```python
from build123d import *

# Parameters (mm, degrees)
SKETCH1_W                       = 22.225
SKETCH1_H                       = 22.225
BOSS_EXTRUDE1_DEPTH             = 38.1
BOSS_EXTRUDE3_REACH             = 43.214
BOSS_EXTRUDE3_DIRECTION_2_REACH = 43.214
SKETCH4_R                       = 2.159
CUT_EXTRUDE1_DEPTH              = 46.486792383
SKETCH8_R                       = 1.5875
CUT_EXTRUDE3_DEPTH              = 8.89
SKETCH7_R                       = 1.5875
CUT_EXTRUDE4_DEPTH              = 8.89
CUT_EXTRUDE6_DEPTH              = 46.486792456
FILLET1_R                       = 0.508
FILLET15_R                      = 1.27
BOSS_EXTRUDE15_DEPTH            = 2.54
SKETCH18_W                      = 10.16
SKETCH18_H                      = 6.120141002
CUT_EXTRUDE7_DEPTH              = 36.83


with BuildPart() as part:
    # Sketch1 → Boss-Extrude1 (new body)
    with BuildSketch(Plane.XY):
        Rectangle(SKETCH1_W, SKETCH1_H)
    extrude(amount=BOSS_EXTRUDE1_DEPTH)

    # Boss-Extrude3: up to this face of the body (flat: up to its plane)
    boss_extrude3_end = Plane(part.part.faces().sort_by_distance((0, 11.1125, 19.05))[0])
    # Sketch3 → Boss-Extrude3 (add, up to the picked face)
    with BuildSketch(Plane(origin=(0, 0, 0), x_dir=(1, 0, 0), z_dir=(0, 1, 0)), mode=Mode.PRIVATE) as boss_extrude3_sk1:
        with BuildLine():
            Line((-11.1125, 0), (11.1125, 0))
            ThreePointArc((11.1125, 0), (0, 11.1125), (-11.1125, 0))
        make_face()
    boss_extrude3_tool1 = split(extrude(boss_extrude3_sk1.sketch, amount=BOSS_EXTRUDE3_REACH, mode=Mode.PRIVATE), bisect_by=boss_extrude3_end, keep=Keep.BOTH, mode=Mode.PRIVATE)
    add(boss_extrude3_tool1.solids().sort_by(Axis((0, 0, -4.716291), (0, 1, 0)))[0])

    # Boss-Extrude3 direction 2: up to this face of the body (flat: up to its plane)
    boss_extrude3_direction_2_end = Plane(part.part.faces().sort_by_distance((0, -11.1125, 19.05))[0])
    # Sketch3 → Boss-Extrude3 direction 2 (add, up to the picked face)
    with BuildSketch(Plane(origin=(0, 0, 0), x_dir=(1, 0, 0), z_dir=(0, 1, 0)), mode=Mode.PRIVATE) as boss_extrude3_direction_2_sk1:
        with BuildLine():
            Line((-11.1125, 0), (11.1125, 0))
            ThreePointArc((11.1125, 0), (0, 11.1125), (-11.1125, 0))
        make_face()
    boss_extrude3_direction_2_tool1 = split(extrude(boss_extrude3_direction_2_sk1.sketch, amount=-BOSS_EXTRUDE3_DIRECTION_2_REACH, mode=Mode.PRIVATE), bisect_by=boss_extrude3_direction_2_end, keep=Keep.BOTH, mode=Mode.PRIVATE)
    add(boss_extrude3_direction_2_tool1.solids().sort_by(Axis((0, 0, -4.716291), (0, -1, 0)))[0])

    # Sketch4 → Cut-Extrude1 (cut, through all)
    with BuildSketch(Plane(origin=(11.1125, 0, 0), x_dir=(0, 0, -1), z_dir=(1, 0, 0))):
        with Locations((-19.05, 0)):
            Circle(SKETCH4_R)
    extrude(amount=-CUT_EXTRUDE1_DEPTH, mode=Mode.SUBTRACT)

    # Sketch8 → Cut-Extrude3 (cut)
    with BuildSketch(Plane(origin=(7.857724106, 0, -7.857724106), x_dir=(-0.7071067811865515, 0, -0.7071067811865436), z_dir=(0.7071067811865436, 0, -0.7071067811865515))):
        Circle(SKETCH8_R)
    extrude(amount=-CUT_EXTRUDE3_DEPTH, mode=Mode.SUBTRACT)

    # Sketch7 → Cut-Extrude4 (cut)
    with BuildSketch(Plane(origin=(-7.857724106, 0, -7.857724106), x_dir=(0.7071067811865512, 0, -0.7071067811865439), z_dir=(0.7071067811865439, 0, 0.7071067811865512))):
        with Locations(Location((0, 0, 0), (0, 0, 180))):
            Circle(SKETCH7_R)
    extrude(amount=CUT_EXTRUDE4_DEPTH, mode=Mode.SUBTRACT)

    # Sketch10 → Cut-Extrude6 (cut, through all)
    with BuildSketch(Plane(origin=(0, -11.1125, 0), x_dir=(-1, 0, 0), z_dir=(0, -1, 0))):
        with BuildLine():
            Line((3.175, -6.35), (3.175, -44.45))
            ThreePointArc((3.175, -44.45), (0, -47.625), (-3.175, -44.45))
            Line((-3.175, -44.45), (-3.175, -6.35))
            ThreePointArc((-3.175, -6.35), (0, -3.175), (3.175, -6.35))
        make_face()
    extrude(amount=-CUT_EXTRUDE6_DEPTH, mode=Mode.SUBTRACT)

    # Fillet1
    fillet1_edges = [part.edges().sort_by_distance(p)[0] for p in [
        (8.89966195, 5e-09, -6.654597918),
        (-6.654597918, -5e-09, -8.89966195),
    ]]
    fillet(fillet1_edges, radius=FILLET1_R)

    # Fillet15
    fillet15_edges = [part.edges().sort_by_distance(p)[0] for p in [
        (-7.14375, -11.1125, 38.1),
        (0, 11.1125, -11.1125),
        (0, -11.1125, -11.1125),
        (-7.14375, 11.1125, 38.1),
        (7.14375, -11.1125, 38.1),
        (-3.175, 11.1125, 22.225),
        (3.175, 11.1125, 22.225),
        (0, 11.1125, 3.175),
        (-3.175, -11.1125, 22.225),
        (0, -11.1125, 3.175),
        (3.175, -11.1125, 22.225),
        (7.14375, 11.1125, 38.1),
        (11.1125, -11.1125, 19.05),
        (-11.1125, -11.1125, 19.05),
        (-11.1125, 11.1125, 19.05),
        (11.1125, 11.1125, 19.05),
    ]]
    fillet(fillet15_edges, radius=FILLET15_R)

    # Sketch14 → Boss-Extrude15 (add, symmetric)
    with BuildSketch(Plane(origin=(0, 0, 0), x_dir=(1, 0, 0), z_dir=(0, 1, 0))):
        Polygon((0.332639056, 2.225283), (-2.103732557, -0.211088613), (0.082871249, -2.397692418), (2.519242862, 0.038679195), align=None)
    extrude(amount=BOSS_EXTRUDE15_DEPTH, both=True)

    # Sketch18 → Cut-Extrude7 (cut)
    with BuildSketch(Plane.XY.offset(38.1)):
        with Locations((0, -11.632570501)):
            Rectangle(SKETCH18_W, SKETCH18_H)
    extrude(amount=-CUT_EXTRUDE7_DEPTH, mode=Mode.SUBTRACT)


solid = part.part
```
Could you check a few things on this model? Use its own coordinates, in mm. A direction names the side the tool comes from. Coordinates: 2 decimals unless noted, no trailing zeros. Loops run counter-clockwise (first coordinate to the right, second up) from the corner with the lowest first, then second, coordinate; pieces in that order, holes last. Notation, with made-up numbers: M 82.25,-8 L 86.25,-8 A20 cw 86.25,15 Z; hole C 60,17 d8. An arc over 180 degrees is marked long. Put each result on its own line as item: value. Start each with the question number.
(1) Suppose I cut it at A-A on z = 19.05. Please give me the cut outline in (x, y) (1 decimal).
(2) Suppose I cut it at C-C on y = 0. Count the separate pieces of the cut face and the enclosed holes in it, then the cut area to 3 significant figures.
(3) I need wall thicknesses on line 1 (X direction, y = -3.75, z = 10) (1 decimal); line 2 (Y direction, x = -5, z = 19.05); line 3 (Y direction, x = 9.25, z = 19.05). Which ranges of each line are inside material? Lowest first, please. Write a range as from..to.
(4) Thinking about a two-plate mould opening in Z: for faces 1 (the face through (-3.175, 1, 22)), 2 (the face through (1.587, 0.022, -1.556)), 3 (the face through (-7, 0, 38.1)), which applies, pulls with the +Z half, pulls with the -Z half, needs draft (parallel to the pull), parting line crosses it, or undercut?
(5) For faces 4 (the face through (-3.557, 10.75, 22.003)), 5 (the face through (-3.5, -8.572, 19.9)), 6 (the face through (7, 0, 38.1)), which set-ups out of +Z, -Z, +X, -X, +Y, -Y let a thin tool reach every point of the face, with its end or its side?
(6) Will these pins go through, and if not, where does the flat tip stop? P1, Ø11, axis at x = 2.5, z = 14.5, coming from the -Y side; P2, Ø4, axis at y = 0, z = 19.05, coming from the +X side; P3, Ø3, axis at x = 3.5, y = -0.5, coming from the -Z side; P4, Ø1, axis at x = -1, y = 0, coming from the -Z side.
Solutions:
1. outline: M -11.1,-9.8 A1.3 ccw -9.8,-11.1 L -5.1,-11.1 L -5.1,-8.6 L -3.2,-8.6 L -3.2,-2.2 L -11.1,-2.2 Z; M -11.1,2.2 L -3.2,2.2 L -3.2,9.8 A1.3 ccw -4.4,11.1 L -9.8,11.1 A1.3 ccw -11.1,9.8 Z; M 3.2,-8.6 L 5.1,-8.6 L 5.1,-11.1 L 9.8,-11.1 A1.3 ccw 11.1,-9.8 L 11.1,-2.2 L 3.2,-2.2 Z; M 3.2,2.2 L 11.1,2.2 L 11.1,9.8 A1.3 ccw 9.8,11.1 L 4.4,11.1 A1.3 ccw 3.2,9.8 Z
2. separate pieces: 3
2. enclosed holes: 0
2. area: 698 mm2
3. line 1: x = -11.1..-3.2, 3.2..11.1
3. line 2: y = -8.57..-2.16, 2.16..11.11
3. line 3: y = -11.11..-2.16, 2.16..11.11
4. face 1: needs draft
4. face 2: undercut
4. face 3: pulls with the +Z half
5. face 4: +Z, +Y
5. face 5: +Z, -Y
5. face 6: +Z, +X, -X, +Y, -Y
6. P1: stops at y = -11.11
6. P2: passes through
6. P3: stops at z = -10.93
6. P4: stops at z = -11.1
